Answer from the drawing. Dimensions are ordinates in mm from the lowest x, y and z of the part. A direction names the side the tool comes from. Give positions to 0.01 mm unless a question says otherwise; leave off trailing zeros. Loops run counter-clockwise (first coordinate to the right, second up) from the corner with the lowest first, then second, coordinate; pieces in that order, holes last. Notation, with made-up numbers: (63.5, -38) - (112.5, -38) arc R12 ccw to (112.5, -31) - close; hole circle Ø4 at (-15, 86.25). An arc over 180 degrees is marked (long way). Answer as CSV lines item,"result". Start each with the question number.
1) Flat-ended cylindrical pins translate along their axes: pin 1 (4.5 mm diameter, centred on x = 8, y = 11.5, fed in from -Z); pin 2 (2.5 mm diameter, centred on y = 3.5, z = 4, fed in from -X); pin 3 (1.6 mm diameter, centred on y = 13.5, z = 4.5, fed in from +X); pin 4 (2 mm diameter, centred on y = 3.5, z = 3, fed in from -X). Find the tip coordinate at first contact, or state that the pin passes through.
2) A cutting plane is placed at C-C (y = 12). Determine the outline of the cut face in (x, z), and give its area (3 significant figures).
3) Find the intervals of material crossed by line 1 along Y through (x, z) = (3.75, 2.5); line 2 along X through (y, z) = (5.25, 4.5); line 3 along Z through (x, y) = (14, 1), in increasing order.
4) For the marked faces 1, 2, 3, 4 and 5, determine the directions among +Z, -Z, +X, -X, +Y, -Y from which every point of the face is accessible in a straight line to the end or side of a thin tool.
5) A cutting plane is placed at A-A (z = 4.5). Determine the outline of the cut face in (x, y).
6) A cutting plane is placed at D-D (y = 6.25). Determine the outline of the cut face in (x, z).
7) A cutting plane is placed at B-B (x = 10.5). Determine the outline of the cut face in (y, z).
8) For a pull along Y with two mould halves and no side action, classify the marked faces 6, 7 and 8 as pulls with the +Y half, pulls with the -Y half, needs draft (parallel to the pull), parting line crosses it, or undercut.
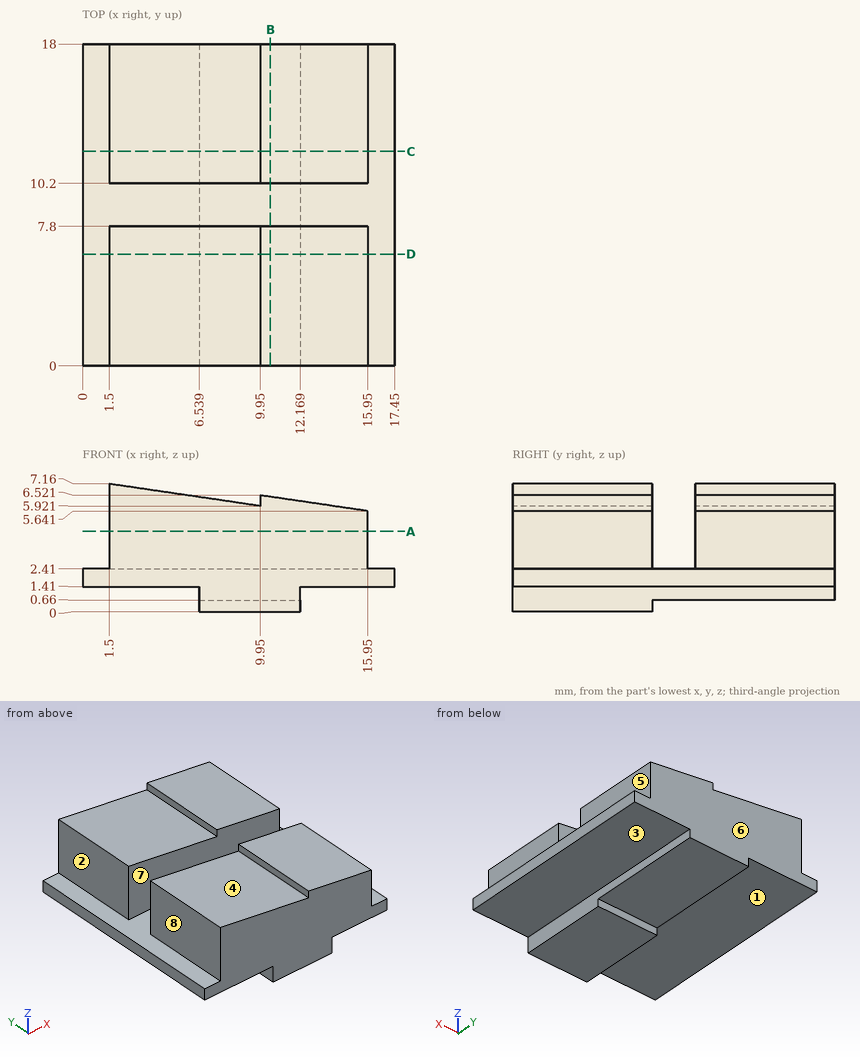
Ans:
1,pin 1,"z = 0.66"
1,pin 2,"x = 1.5"
1,pin 3,"x = 15.95"
1,pin 4,"x = 0"
2,outline,"(0, 1.41) - (6.54, 1.41) - (6.54, 0.66) - (12.17, 0.66) - (12.17, 1.41) - (17.45, 1.41) - (17.45, 2.41) - (15.95, 2.41) - (15.95, 5.64) - (9.95, 6.52) - (9.95, 5.92) - (1.5, 7.16) - (1.5, 2.41) - (0, 2.41) - close"
2,area,"78.6 mm2"
3,line 1,"0 to 7.8, 10.2 to 18"
3,line 2,"1.5 to 15.95"
3,line 3,"1.41 to 5.93"
4,face 1,"-Z, -X, +Y, -Y"
4,face 2,"+Z, -X, +Y, -Y"
4,face 3,"-Z, +X, +Y, -Y"
4,face 4,"+Z, +Y, -Y"
4,face 5,"+Z, +X, +Y, -Y"
5,outline,"(1.5, 0) - (15.95, 0) - (15.95, 7.8) - (1.5, 7.8) - close; (1.5, 10.2) - (15.95, 10.2) - (15.95, 18) - (1.5, 18) - close"
6,outline,"(0, 1.41) - (6.54, 1.41) - (6.54, 0) - (12.17, 0) - (12.17, 1.41) - (17.45, 1.41) - (17.45, 2.41) - (15.95, 2.41) - (15.95, 5.64) - (9.95, 6.52) - (9.95, 5.92) - (1.5, 7.16) - (1.5, 2.41) - (0, 2.41) - close"
7,outline,"(0, 0) - (7.8, 0) - (7.8, 0.66) - (18, 0.66) - (18, 6.44) - (10.2, 6.44) - (10.2, 2.41) - (7.8, 2.41) - (7.8, 6.44) - (0, 6.44) - close"
8,face 6,"pulls with the +Y half"
8,face 7,"undercut"
8,face 8,"needs draft"
